from build123d import *

# Parameters (mm, degrees)
BOSS_EXTRUDE1_DEPTH     = 5
FILLET1_R               = 10
FILLET2_R               = 10
FILLET3_R               = 10
FILLET4_R               = 10
SKETCH2_W               = 5
SKETCH2_H               = 7.5
BOSS_EXTRUDE2_DEPTH     = 25
MIRROR2_COPY_1_SKETCH_W = 5
MIRROR2_COPY_1_SKETCH_H = 7.5
MIRROR2_COPY_1_DEPTH    = 25
SKETCH3_R               = 1.5
CUT_EXTRUDE1_DEPTH      = 119.966907163
SKETCH4_W               = 2.694155106
SKETCH4_H               = 50
SKETCH4_W_2             = 3
BOSS_EXTRUDE3_DEPTH     = 8
SKETCH5_W               = 5.694155106
SKETCH5_H               = 3
CUT_EXTRUDE2_DEPTH      = 42
CUT_EXTRUDE3_DEPTH      = 115.422257996
FILLET5_R               = 10
FILLET6_R               = 10
FILLET7_R               = 10
FILLET8_R               = 10
BOSS_EXTRUDE4_REACH     = 112.848
SKETCH7_W               = 5
SKETCH7_H               = 5
FILLET9_R               = 10
FILLET10_DEPTH          = 5
FILLET11_R              = 10
FILLET12_DEPTH          = 5
FILLET13_R              = 2


with BuildPart() as part:
    # Sketch1 → Boss-Extrude1 (new body)
    with BuildSketch(Plane(origin=(0, 0, 0), x_dir=(1, 0, 0), z_dir=(0, 1, 0))):
        with BuildLine():
            Line((-34.25, 15.75), (-26.75, 15.75))
            Line((-26.75, 15.75), (-26.75, 18.25))
            ThreePointArc((-26.75, 18.25), (-27.633883476, 20.383883476), (-25.5, 19.5))
            Line((-25.5, 19.5), (25.5, 19.5))
            ThreePointArc((25.5, 19.5), (26.75, 20.75), (28, 19.5))
            ThreePointArc((28, 19.5), (27.633883476, 18.616116524), (26.75, 18.25))
            Line((26.75, 18.25), (26.75, 15.75))
            Line((26.75, 15.75), (34.25, 15.75))
            Line((34.25, 15.75), (58.875, 15.75))
            Line((58.875, 15.75), (58.875, 23.25))
            Line((58.875, 23.25), (-58.875, 23.25))
            Line((-58.875, 23.25), (-58.875, 15.75))
            Line((-58.875, 15.75), (-34.25, 15.75))
        make_face()
        with BuildLine():
            Line((-26.75, 18.25), (-26.75, 15.75))
            Line((-26.75, 15.75), (-15.25, 15.75))
            Line((-15.25, 15.75), (15.25, 15.75))
            Line((15.25, 15.75), (26.75, 15.75))
            Line((26.75, 15.75), (26.75, 18.25))
            ThreePointArc((26.75, 18.25), (25.866116524, 18.616116524), (25.5, 19.5))
            Line((25.5, 19.5), (-25.5, 19.5))
            ThreePointArc((-25.5, 19.5), (-25.866116524, 18.616116524), (-26.75, 18.25))
        make_face()
        with BuildLine():
            Line((0, -19.5), (-25.5, -19.5))
            ThreePointArc((-25.5, -19.5), (-26.75, -20.75), (-28, -19.5))
            Line((-28, -19.5), (-58.875, -19.5))
            Line((-58.875, -19.5), (-58.875, -23.25))
            Line((-58.875, -23.25), (58.875, -23.25))
            Line((58.875, -23.25), (58.875, -15.75))
            Line((58.875, -15.75), (34.25, -15.75))
            Line((34.25, -15.75), (26.75, -15.75))
            Line((26.75, -15.75), (26.75, -18.25))
            ThreePointArc((26.75, -18.25), (27.633883476, -18.616116524), (28, -19.5))
            ThreePointArc((28, -19.5), (26.75, -20.75), (25.5, -19.5))
            Line((25.5, -19.5), (0, -19.5))
        make_face()
        with BuildLine():
            Line((-26.75, -15.75), (-26.75, -18.25))
            ThreePointArc((-26.75, -18.25), (-25.866116524, -18.616116524), (-25.5, -19.5))
            Line((-25.5, -19.5), (0, -19.5))
            Line((0, -19.5), (25.5, -19.5))
            ThreePointArc((25.5, -19.5), (25.866116524, -18.616116524), (26.75, -18.25))
            Line((26.75, -18.25), (26.75, -15.75))
            Line((26.75, -15.75), (15.25, -15.75))
            Line((15.25, -15.75), (-15.25, -15.75))
            Line((-15.25, -15.75), (-26.75, -15.75))
        make_face()
        with BuildLine():
            ThreePointArc((-28, -19.5), (-27.633883476, -18.616116524), (-26.75, -18.25))
            Line((-26.75, -18.25), (-26.75, -15.75))
            Line((-26.75, -15.75), (-34.25, -15.75))
            Line((-34.25, -15.75), (-58.875, -15.75))
            Line((-58.875, -15.75), (-58.875, -19.5))
            Line((-58.875, -19.5), (-28, -19.5))
        make_face()
        Polygon((-26.75, 0), (-26.75, -15.75), (-15.25, -15.75), (-15.25, 0), (-15.25, 15.75), (-26.75, 15.75), align=None)
        Polygon((15.25, 0), (15.25, -15.75), (26.75, -15.75), (26.75, 15.75), (15.25, 15.75), align=None)
    extrude(amount=BOSS_EXTRUDE1_DEPTH)

    # Fillet1
    fillet1_edges = [part.edges().sort_by_distance(p)[0] for p in [
        (-26.75, 2.5, -15.75),
    ]]
    fillet(fillet1_edges, radius=FILLET1_R)

    # Fillet2
    fillet2_edges = [part.edges().sort_by_distance(p)[0] for p in [
        (-26.75, 2.5, 15.75),
    ]]
    fillet(fillet2_edges, radius=FILLET2_R)

    # Fillet3
    fillet3_edges = [part.edges().sort_by_distance(p)[0] for p in [
        (26.75, 2.5, -15.75),
    ]]
    fillet(fillet3_edges, radius=FILLET3_R)

    # Fillet4
    fillet4_edges = [part.edges().sort_by_distance(p)[0] for p in [
        (26.75, 2.5, 15.75),
    ]]
    fillet(fillet4_edges, radius=FILLET4_R)

    # Sketch2 → Boss-Extrude2 (add)
    with BuildSketch(Plane(origin=(0, 5, 0), x_dir=(1, 0, 0), z_dir=(0, 1, 0))):
        with Locations((56.375, 19.5)):
            Rectangle(SKETCH2_W, SKETCH2_H)
    boss_extrude2 = extrude(amount=BOSS_EXTRUDE2_DEPTH)

    # Mirror1: Boss-Extrude2 across plane
    add(boss_extrude2.mirror(Plane(origin=(0, 0, 0), x_dir=(0, 0, 1), z_dir=(1, 0, 0))))

    # Mirror2: Boss-Extrude2 across plane
    add(boss_extrude2.mirror(Plane.XY))

    # Mirror2 copy 1 sketch → Mirror2 copy 1 (add)
    with BuildSketch(Plane(origin=(0, 5, 0), x_dir=(-1, 0, 0), z_dir=(0, 1, 0))):
        with Locations((56.375, 19.5)):
            Rectangle(MIRROR2_COPY_1_SKETCH_W, MIRROR2_COPY_1_SKETCH_H)
    extrude(amount=MIRROR2_COPY_1_DEPTH)

    # Sketch3 → Cut-Extrude1 (cut, symmetric)
    with BuildSketch(Plane.ZY.offset(-53.875)):
        with Locations((-19.5, 27)):
            Circle(SKETCH3_R)
    cut_extrude1 = extrude(amount=CUT_EXTRUDE1_DEPTH, both=True, mode=Mode.SUBTRACT)

    # Mirror3: Cut-Extrude1 across plane
    add(cut_extrude1.mirror(Plane.XY), mode=Mode.SUBTRACT)

    # Sketch4 → Boss-Extrude3 (add)
    with BuildSketch(Plane(origin=(0, 0, 0), x_dir=(-1, 0, 0), z_dir=(0, -1, 0))):
        with Locations((-28.097077553, -48.25)):
            Rectangle(SKETCH4_W, SKETCH4_H)
        with Locations((-25.25, -48.25)):
            Rectangle(SKETCH4_W_2, SKETCH4_H)
    boss_extrude3 = extrude(amount=-BOSS_EXTRUDE3_DEPTH)

    # Sketch5 → Cut-Extrude2 (cut)
    with BuildSketch(Plane(origin=(0, 0, 23.25), x_dir=(-1, 0, 0), z_dir=(0, 0, -1))):
        with Locations((-26.597077553, 6.5)):
            Rectangle(SKETCH5_W, SKETCH5_H)
    cut_extrude2 = extrude(amount=-CUT_EXTRUDE2_DEPTH, mode=Mode.SUBTRACT)

    # Sketch6 → Cut-Extrude3 (cut, through all)
    with BuildSketch(Plane.ZY.offset(-23.75)):
        with BuildLine():
            ThreePointArc((71.25, 4), (70.664213562, 5.414213562), (69.25, 6))
            Line((69.25, 6), (69.25, 2))
            ThreePointArc((69.25, 2), (70.664213562, 2.585786438), (71.25, 4))
        make_face()
        with BuildLine():
            Line((69.25, 2), (69.25, 6))
            ThreePointArc((69.25, 6), (67.25, 4), (69.25, 2))
        make_face()
    cut_extrude3 = extrude(amount=-CUT_EXTRUDE3_DEPTH, mode=Mode.SUBTRACT)

    # Fillet5
    fillet5_edges = [part.edges().sort_by_distance(p)[0] for p in [
        (23.75, 2.5, 23.25),
    ]]
    fillet(fillet5_edges, radius=FILLET5_R)

    # Fillet6
    fillet6_edges = [part.edges().sort_by_distance(p)[0] for p in [
        (29.444155106, 2.5, 23.25),
    ]]
    fillet(fillet6_edges, radius=FILLET6_R)

    # Mirror4: Boss-Extrude3, Cut-Extrude2, Cut-Extrude3 across plane
    add(boss_extrude3.mirror(Plane(origin=(0, 0, 0), x_dir=(0, 0, 1), z_dir=(1, 0, 0))))
    add(cut_extrude2.mirror(Plane(origin=(0, 0, 0), x_dir=(0, 0, 1), z_dir=(1, 0, 0))), mode=Mode.SUBTRACT)
    add(cut_extrude3.mirror(Plane(origin=(0, 0, 0), x_dir=(0, 0, 1), z_dir=(1, 0, 0))), mode=Mode.SUBTRACT)

    # Fillet7
    fillet7_edges = [part.edges().sort_by_distance(p)[0] for p in [
        (-23.75, 2.5, 23.25),
    ]]
    fillet(fillet7_edges, radius=FILLET7_R)

    # Fillet8
    fillet8_edges = [part.edges().sort_by_distance(p)[0] for p in [
        (-29.444155106, 2.5, 23.25),
    ]]
    fillet(fillet8_edges, radius=FILLET8_R)

    # Sketch7 → Boss-Extrude4 (add, up to next)
    with BuildSketch(Plane.XY.offset(-15.75), mode=Mode.PRIVATE) as boss_extrude4_sk1:
        with Locations((-56.375, 2.5)):
            Rectangle(SKETCH7_W, SKETCH7_H)
    boss_extrude4_tool1 = extrude(boss_extrude4_sk1.sketch, amount=BOSS_EXTRUDE4_REACH, mode=Mode.PRIVATE) - part.part
    boss_extrude4 = boss_extrude4_tool1.solids().sort_by_distance((-56.375, 2.5, -15.75))[0]
    add(boss_extrude4)

    # Mirror5: Boss-Extrude4 across plane
    add(boss_extrude4.mirror(Plane(origin=(0, 0, 0), x_dir=(0, 0, 1), z_dir=(1, 0, 0))))

    # Fillet9
    # the kernel refuses this fillet: 10 mm, written as the material it adds along each edge
    with BuildSketch(Plane(origin=(53.875, 0, -15.75), x_dir=(0, 0, 1), z_dir=(0, 1, 0))) as fillet9_piece_1:
        with BuildLine():
            CenterArc((FILLET9_R, -FILLET9_R), FILLET9_R, 90, 90)
            Line((0, -FILLET9_R), (0, 0))
            Line((0, 0), (FILLET9_R, 0))
        make_face()
    extrude(amount=5)

    # Fillet10: read off the stored shape, not the designer's step
    # Fillet10 outline → Fillet10 (add)
    with BuildSketch(Plane(origin=(0, 0, 0), x_dir=(1, 0, 0), z_dir=(0, 1, 0))):
        with BuildLine():
            ThreePointArc((53.875, -5.75), (50.946067812, -12.821067812), (43.875, -15.75))
            Line((43.875, -15.75), (53.875, -15.75))
            Line((53.875, -15.75), (53.875, -5.75))
        make_face()
    extrude(amount=FILLET10_DEPTH)

    # Fillet11
    # the kernel refuses this fillet: 10 mm, written as the material it adds along each edge
    with BuildSketch(Plane(origin=(-53.875, 0, -15.75), x_dir=(1, 0, 0), z_dir=(0, 1, 0))) as fillet11_piece_1:
        with BuildLine():
            CenterArc((FILLET11_R, -FILLET11_R), FILLET11_R, 90, 90)
            Line((0, -FILLET11_R), (0, 0))
            Line((0, 0), (FILLET11_R, 0))
        make_face()
    extrude(amount=5)

    # Fillet12: read off the stored shape, not the designer's step
    # Fillet12 outline → Fillet12 (add)
    with BuildSketch(Plane(origin=(0, 0, 0), x_dir=(1, 0, 0), z_dir=(0, 1, 0))):
        with BuildLine():
            Line((-53.875, -15.75), (-43.875, -15.75))
            ThreePointArc((-43.875, -15.75), (-50.946067812, -12.821067812), (-53.875, -5.75))
            Line((-53.875, -5.75), (-53.875, -15.75))
        make_face()
    extrude(amount=FILLET12_DEPTH)

    # Fillet13
    fillet13_edges = [part.edges().sort_by_distance(p)[0] for p in [
        (0, 0, 23.25),
        (23.75, 0, 53.25),
        (20.821067812, 0, 26.178932188),
        (29.444155106, 0, 53.25),
        (32.373087294, 0, 26.178932188),
        (-26.597077553, 0, 73.25),
        (-58.875, 0, 0),
        (0, 0, -23.25),
        (58.875, 0, 0),
        (-23.75, 0, 53.25),
        (-20.821067812, 0, 26.178932188),
        (-49.159577553, 0, 23.25),
        (-29.444155106, 0, 53.25),
        (-32.373087294, 0, 26.178932188),
        (49.159577553, 0, 23.25),
    ]]
    fillet(fillet13_edges, radius=FILLET13_R - 0.0001)  # a hair under: the kernel refuses the full size


solid = part.part
Could you check a few things on this model? Use its own coordinates, in mm. A direction names the side the tool comes from. Give positions to 0.01 mm unless a question says otherwise; leave off trailing zeros. Order: outer loops, then holes, each group sorted by start corner. A loop starts at its lowest first (then second) coordinate and runs counter-clockwise, first axis right, second up. Notation, with made-up numbers: (-32, 2) -> (-14, 2) arc R10 cw to (-14, 6) -> close; hole circle Ø2 at (51.5, 19.5). An arc over 180 degrees is marked (long way). Return JSON: item names as keys, results as strings.
1. On a 3-axis mill with a long thin cutter (end or side, diameter ignored), from which of +Z, -Z, +X, -X, +Y, -Y can I reach the whole of each face in a straight line? I mean faces 1 (the flat face through (-53.875, 17, -19)), 2 (the flat face through (56, 17, 15.75)), 3 (the cylindrical face through (-50.868, 2.465, 12.898)). Say none if no direction works.
Answer list:
{"face 1": "+Z, -Z, +Y", "face 2": "+X, -X, +Y", "face 3": "+Y, -Y"}
2. Imagine slicing it at A-A on x = -10. List the corners of the cut face in (y, z) for me, then the cut area to 3 significant figures.
Answer list:
{"outline": "(0, -21.25) arc R2 ccw to (2, -23.25) -> (5, -23.25) -> (5, -15.75) -> (0, -15.75) -> close; (0, 15.75) -> (5, 15.75) -> (5, 23.25) -> (2, 23.25) arc R2 ccw to (0, 21.25) -> close", "area": "73.3 mm2"}
3. Imagine slicing it at D-D on y = 27. Give the number of separate pieces and of enclosed holes in the cut face, then the cut area to 3 significant figures.
Answer list:
{"separate pieces": "8", "enclosed holes": "0", "area": "90.0 mm2"}
4. Thinking about a two-plate mould opening in X: for faces 4 (the cylindrical face through (-29.76, 2.54, -12.9)), 5 (the flat face through (-1, 5, 20)), 6 (the flat face through (58.875, 3, -5)), 7 (the flat face through (-56, 17, -15.75)), which applies, pulls with the +X half, pulls with the -X half, needs draft (parallel to the pull), parting line crosses it, or undercut?
Answer list:
{"face 4": "undercut", "face 5": "undercut", "face 6": "pulls with the +X half", "face 7": "needs draft"}
5. Imagine slicing it at B-B on y = 10.5. List the corners of the cut face in (x, z) for me (3 decimals).
Answer list:
{"outline": "(-58.875, -23.25) -> (-53.875, -23.25) -> (-53.875, -15.75) -> (-58.875, -15.75) -> close; (-58.875, 15.75) -> (-53.875, 15.75) -> (-53.875, 23.25) -> (-58.875, 23.25) -> close; (53.875, -23.25) -> (58.875, -23.25) -> (58.875, -15.75) -> (53.875, -15.75) -> close; (53.875, 15.75) -> (58.875, 15.75) -> (58.875, 23.25) -> (53.875, 23.25) -> close"}
6. I need wall thicknesses on line 1 (X direction, y = 1.9, z = -19.5); line 2 (Y direction, x = -55.35, z = -19.5); line 3 (X direction, y = 1.75, z = 46). Which ranges of each line are inside material? Lowest first, please. Write a range as from..to.
Answer list:
{"line 1": "x = -58.87..-28, -25.5..25.5, 28..58.87", "line 2": "y = 0..25.5, 28.5..30", "line 3": "x = -29.43..-23.77, 23.77..29.43"}
7. For pin 1 Ø2.5 at (x, y) = (-57.5, 22.5) entering from +Z; pin 2 Ø1.5 at (x, y) = (-28, 6.5) entering from -Z; pin 3 Ø6.5 at (x, z) = (-27.5, 70) entering from +Y, each with a flat end and sliding along its axis, tell me the tip position at first contact or that it passes through.
Answer list:
{"pin 1": "stops at z = 23.25", "pin 2": "stops at z = 65.25", "pin 3": "stops at y = 8"}
8. Imagine slicing it at C-C on z = -4. List the corners of the cut face in (x, y) for me (3 decimals).
Answer list:
{"outline": "(-58.875, 2) arc R2 ccw to (-56.875, 0) -> (-53.875, 0) -> (-53.875, 5) -> (-58.875, 5) -> close; (-26.75, 0) -> (-15.25, 0) -> (-15.25, 5) -> (-26.75, 5) -> close; (15.25, 0) -> (26.75, 0) -> (26.75, 5) -> (15.25, 5) -> close; (53.875, 0) -> (56.875, 0) arc R2 ccw to (58.875, 2) -> (58.875, 5) -> (53.875, 5) -> close"}
